Design review of the part built by this model. Coordinates are the model's own, in mm. Face numbers are marked on the shaded views. A direction names the side the tool comes from. Coordinates: 2 decimals unless noted, no trailing zeros. Loops run counter-clockwise (first coordinate to the right, second up) from the corner with the lowest first, then second, coordinate; pieces in that order, holes last. Notation, with made-up numbers: M -32.5,-36 L 26.5,-36 A31 ccw 26.5,-2 Z; hole C 86,82.5 d2. An arc over 180 degrees is marked long. One line per item, written item: value.
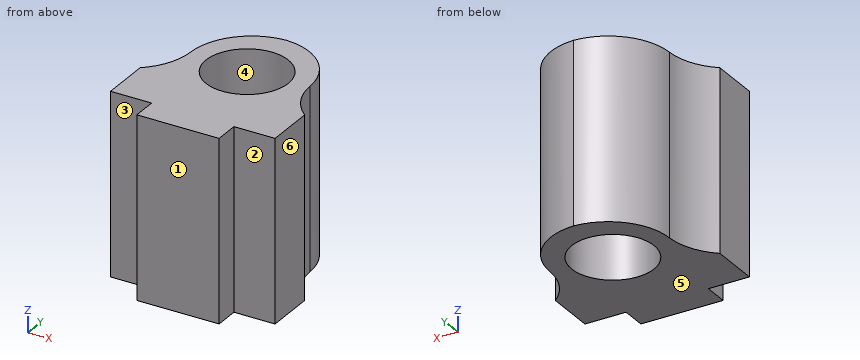
```python
from build123d import *

# Parameters (mm, degrees)
SKETCH6_W           = 20
SKETCH6_H           = 22
BOSS_EXTRUDE5_DEPTH = 6
SKETCH7_W           = 10
SKETCH7_H           = 22
BOSS_EXTRUDE6_DEPTH = 3
SKETCH8_W           = 14.5
SKETCH8_H           = 22
BOSS_EXTRUDE7_DEPTH = 13
SKETCH9_R           = 5
CUT_EXTRUDE1_DEPTH  = 36.284557529
FILLET1_R           = 7.5
FILLET2_R           = 7.5


with BuildPart() as part:
    # Sketch6 → Boss-Extrude5 (new body)
    with BuildSketch(Plane(origin=(0, 0, 0), x_dir=(1, 0, 0), z_dir=(0, 1, 0))):
        with Locations((10, 11)):
            Rectangle(SKETCH6_W, SKETCH6_H)
    extrude(amount=BOSS_EXTRUDE5_DEPTH)

    # Sketch7 → Boss-Extrude6 (add)
    with BuildSketch(Plane.XZ):
        with Locations((10, -11)):
            Rectangle(SKETCH7_W, SKETCH7_H)
    extrude(amount=BOSS_EXTRUDE6_DEPTH)

    # Sketch8 → Boss-Extrude7 (add)
    with BuildSketch(Plane(origin=(0, 6, 0), x_dir=(1, 0, 0), z_dir=(0, 1, 0))):
        with Locations((10, 11)):
            Rectangle(SKETCH8_W, SKETCH8_H)
    extrude(amount=BOSS_EXTRUDE7_DEPTH)

    # Sketch9 → Cut-Extrude1 (cut, through all)
    with BuildSketch(Plane.XY):
        with Locations((10, 11)):
            Circle(SKETCH9_R)
    extrude(amount=-CUT_EXTRUDE1_DEPTH, mode=Mode.SUBTRACT)

    # Fillet1
    # the kernel refuses this fillet: 7.5 mm, written as the material it takes off along each edge
    with BuildSketch(Plane(origin=(17.25, 19, -40.75), x_dir=(-1, 0, 0), z_dir=(0, 0, 1))) as fillet1_piece_1:
        with BuildLine():
            CenterArc((FILLET1_R, FILLET1_R), FILLET1_R, 180, 90)
            Line((0, FILLET1_R), (0, 0))
            Line((0, 0), (FILLET1_R, 0))
        make_face()
    extrude(amount=59.5, mode=Mode.SUBTRACT)
    with BuildSketch(Plane(origin=(2.75, 19, 18.75), x_dir=(0, -1, 0), z_dir=(0, 0, -1))) as fillet1_piece_2:
        with BuildLine():
            CenterArc((FILLET1_R, -FILLET1_R), FILLET1_R, 90, 90)
            Line((0, -FILLET1_R), (0, 0))
            Line((0, 0), (FILLET1_R, 0))
        make_face()
    extrude(amount=59.5, mode=Mode.SUBTRACT)

    # Fillet2
    # the kernel refuses this fillet: 7.5 mm, written as the material it adds along each edge
    with BuildSketch(Plane(origin=(17.25, 6, -22), x_dir=(1, 0, 0), z_dir=(0, 0, 1))) as fillet2_piece_1:
        with BuildLine():
            CenterArc((7.496865043, 5.806657581), FILLET2_R, 181.171427285, 49.563032728)
            Line((-0.001567478, 5.65332879), (-0.75141073, 5.637995911))
            ThreePointArc((-0.75141073, 5.637995911), (-0.75, 5.5), (-0.75, 0))
            Line((-0.75, 0), (0, -0.75))
            ThreePointArc((0, -0.75), (1.375, -0.75), (2.275313496, -0.580665758))
            Line((2.275313496, -0.580665758), (2.75, 0))
        make_face()
    extrude(amount=22)
    with BuildSketch(Plane(origin=(2.75, 6, 0), x_dir=(0.00027726642617420565, 0.9999999615616638, 0), z_dir=(0, 0, -1))) as fillet2_piece_2:
        with BuildLine():
            CenterArc((5.804578729, -7.498474746), FILLET2_R, 91.155541089, 49.563032728)
            Line((-0.000762483, -2.749999894), (-0.581296604, -2.275152409))
            ThreePointArc((-0.581296604, -2.275152409), (-0.750381213, -1.374791997), (-0.749999971, 0.00020795))
            Line((-0.749999971, 0.00020795), (0.00020795, 0.749999971))
            ThreePointArc((0.00020795, 0.749999971), (5.500207738, 0.748475006), (5.638204036, 0.749847475))
            Line((5.638204036, 0.749847475), (5.653329008, 0))
        make_face()
    extrude(amount=22)


solid = part.part
```
(1) Insertion check: pin 1 (1.5 mm diameter, centred on x = 2.5, z = -11.5, fed in from -Y); pin 2 (4 mm diameter, centred on y = 10.5, z = -10, fed in from -X); pin 3 (1 mm diameter, centred on x = 11.5, z = -8, fed in from +Y). Each pin has a flat end and moves straight along its axis. Give the tip position at first contact, or say it passes through.
Reply:
pin 1: stops at y = 0
pin 2: stops at x = 1.98
pin 3: stops at y = 18.9
(2) Mouldability with a two-part tool opening along X and no side actions: class the marked faces 4, 5 and 6 as released by +X, released by -X, zero draft, split by the parting line, or undercut.
Reply:
face 4: undercut
face 5: zero draft
face 6: released by +X
(3) We need section B-B on y = 10.5. State the section outline as (x, z) points, then the cut area to 3 significant figures.
Reply:
outline: M 2.64,-22 L 5.03,-22 L 5.03,0 L 2.64,0 Z; M 14.97,-22 L 17.36,-22 L 17.36,0 L 14.97,0 Z
area: 105 mm2
(4) We need section C-C on x = 10.5. State the section outline as (y, z) points, then the cut area to 3 significant figures.
Reply:
outline: M -3,-22 L 6.03,-22 L 6.03,0 L -3,0 Z; M 15.97,-22 L 18.96,-22 L 18.96,0 L 15.97,0 Z
area: 264 mm2
(5) Tool access review of the marked faces 1, 2 and 3: name each direction out of +Z, -Z, +X, -X, +Y, -Y from which nothing blocks a thin tool from reaching the whole face with its end or side.
Reply:
face 1: +Z, -Z, +X, -X, -Y
face 2: +Z, -Z, +X, -Y
face 3: +Z, -Z, -X, -Y
(6) We need section A-A on z = -7.75. State the section outline as (x, y) points.
Reply:
outline: M 0,0 L 5,0 L 5,-3 L 15,-3 L 15,0 L 20,0 L 20,6 A7.5 cw 17.25,11.65 A7.5 ccw 10,19 A7.5 ccw 2.75,11.65 A7.5 cw 0,6 Z; hole C 10,11 d10
(7) We need section D-D on y = -0.75. State the section outline as (x, z) points.
Reply:
outline: M 5,-22 L 15,-22 L 15,0 L 5,0 Z
(8) To check wall thickness, follow line 1 along Y through (x, z) = (10, -9.5); line 2 along X through (y, z) = (-1, -6); line 3 along X through (y, z) = (10, -17.5). State the ranges of each line that lie inside material, in increasing order. Write a range as [from, to].
Reply:
line 1: y = [-3, 6], [16, 19]
line 2: x = [5, 15]
line 3: x = [2.53, 5.1], [14.9, 17.47]
